Verification items for the finished model (mm, model axes). Coordinates: 2 decimals unless noted, no trailing zeros. Write each loop counter-clockwise with the first axis right and the second up, starting at its lowest first coordinate (ties: lowest second). Pieces come first, ordered by that corner, then holes. Notation, with made-up numbers: (33.5, 21) -> (51.5, 21) arc R17 ccw to (51.5, 48) -> close; hole circle Ø4 at (3.5, 85). An arc over 180 degrees is marked (long way). Answer in a Markdown table with one row per item.
```python
from build123d import *

# Parameters (mm, degrees)
SKETCH1_W               = 127
SKETCH1_H               = 101.6
BOSS_EXTRUDE1_DEPTH     = 3.175
CUT_EXTRUDE3_DEPTH      = 3.175
SKETCH4_W               = 6.35
SKETCH4_H               = 10.16
CUT_EXTRUDE4_DEPTH      = 3.175
MIRROR4_COPY_1_SKETCH_W = 6.35
MIRROR4_COPY_1_SKETCH_H = 10.16
MIRROR4_COPY_1_DEPTH    = 3.175


with BuildPart() as part:
    # Sketch1 → Boss-Extrude1 (new body)
    with BuildSketch(Plane(origin=(0, 0, 0), x_dir=(0, 0, -1), z_dir=(1, 0, 0))):
        Polygon((-127, -101.6), (-127, -155.575), (-114.3, -155.575), (-114.3, -152.4), (-101.6, -152.4), (-101.6, -155.575), (-88.9, -155.575), (-88.9, -152.4), (-76.2, -152.4), (-76.2, -155.575), (-63.5, -155.575), (-63.5, -101.6), (63.5, -101.6), (63.5, -155.575), (76.2, -155.575), (76.2, -152.4), (88.9, -152.4), (88.9, -155.575), (101.6, -155.575), (101.6, -152.4), (114.3, -152.4), (114.3, -155.575), (127, -155.575), (127, -101.6), (133.35, -101.6), (133.35, -50.8), (127, -50.8), (127, 50.8), (133.35, 50.8), (133.35, 101.6), (127, 101.6), (127, 155.575), (114.3, 155.575), (114.3, 152.4), (101.6, 152.4), (101.6, 155.575), (88.9, 155.575), (88.9, 152.4), (76.2, 152.4), (76.2, 155.575), (63.5, 155.575), (63.5, 101.6), (-63.5, 101.6), (-63.5, 155.575), (-76.2, 155.575), (-76.2, 152.4), (-88.9, 152.4), (-88.9, 155.575), (-101.6, 155.575), (-101.6, 152.4), (-114.3, 152.4), (-114.3, 155.575), (-127, 155.575), (-127, 101.6), (-133.35, 101.6), (-133.35, 50.8), (-127, 50.8), (-127, -50.8), (-133.35, -50.8), (-133.35, -101.6), align=None)
        Rectangle(SKETCH1_W, SKETCH1_H, mode=Mode.SUBTRACT)
    extrude(amount=BOSS_EXTRUDE1_DEPTH)

    # Sketch3 → Cut-Extrude3 (cut)
    with BuildSketch(Plane(origin=(3.175, 0, 0), x_dir=(0, 0, -1), z_dir=(1, 0, 0))):
        with BuildLine():
            Line((1.060660172, 84.639339828), (0, 85.7))
            Line((0, 85.7), (-1.060660172, 84.639339828))
            ThreePointArc((-1.060660172, 84.639339828), (0, 84.2), (1.060660172, 84.639339828))
        make_face()
        with BuildLine():
            Line((-1.060660172, 84.639339828), (0, 85.7))
            Line((0, 85.7), (1.060660172, 84.639339828))
            ThreePointArc((1.060660172, 84.639339828), (1.385819299, 85.125974851), (1.5, 85.7))
            ThreePointArc((1.5, 85.7), (-0.574025149, 87.085819299), (-1.060660172, 84.639339828))
        make_face()
        with BuildLine():
            ThreePointArc((1.060660172, 67.760660172), (0, 68.2), (-1.060660172, 67.760660172))
            Line((-1.060660172, 67.760660172), (0, 66.7))
            Line((0, 66.7), (1.060660172, 67.760660172))
        make_face()
        with BuildLine():
            Line((0, 66.7), (-1.060660172, 67.760660172))
            ThreePointArc((-1.060660172, 67.760660172), (-0.574025149, 65.314180701), (1.5, 66.7))
            ThreePointArc((1.5, 66.7), (1.385819299, 67.274025149), (1.060660172, 67.760660172))
            Line((1.060660172, 67.760660172), (0, 66.7))
        make_face()
        with BuildLine():
            ThreePointArc((11, 76.2), (10.074025149, 77.585819299), (8.439339828, 77.260660172))
            Line((8.439339828, 77.260660172), (9.5, 76.2))
            Line((9.5, 76.2), (8.439339828, 75.139339828))
            ThreePointArc((8.439339828, 75.139339828), (10.074025149, 74.814180701), (11, 76.2))
        make_face()
        with BuildLine():
            Line((9.5, 76.2), (8.439339828, 77.260660172))
            ThreePointArc((8.439339828, 77.260660172), (8, 76.2), (8.439339828, 75.139339828))
            Line((8.439339828, 75.139339828), (9.5, 76.2))
        make_face()
        with BuildLine():
            ThreePointArc((-8, 76.2), (-8.114180701, 76.774025149), (-8.439339828, 77.260660172))
            Line((-8.439339828, 77.260660172), (-9.5, 76.2))
            Line((-9.5, 76.2), (-8.439339828, 75.139339828))
            ThreePointArc((-8.439339828, 75.139339828), (-8.114180701, 75.625974851), (-8, 76.2))
        make_face()
        with BuildLine():
            Line((-9.5, 76.2), (-8.439339828, 77.260660172))
            ThreePointArc((-8.439339828, 77.260660172), (-11, 76.2), (-8.439339828, 75.139339828))
            Line((-8.439339828, 75.139339828), (-9.5, 76.2))
        make_face()
    extrude(amount=-CUT_EXTRUDE3_DEPTH, mode=Mode.SUBTRACT)

    # Sketch4 → Cut-Extrude4 (cut)
    with BuildSketch(Plane(origin=(3.175, 0, 0), x_dir=(0, 0, -1), z_dir=(1, 0, 0))):
        with Locations((130.175, 86.36)):
            Rectangle(SKETCH4_W, SKETCH4_H)
        with Locations((130.175, 66.04)):
            Rectangle(SKETCH4_W, SKETCH4_H)
    cut_extrude4 = extrude(amount=-CUT_EXTRUDE4_DEPTH, mode=Mode.SUBTRACT)

    # Mirror3: Cut-Extrude4 across plane
    add(cut_extrude4.mirror(Plane.ZX), mode=Mode.SUBTRACT)

    # Mirror4: Cut-Extrude4 across plane
    add(cut_extrude4.mirror(Plane.XY), mode=Mode.SUBTRACT)

    # Mirror4 copy 1 sketch → Mirror4 copy 1 (cut)
    with BuildSketch(Plane(origin=(3.175, 0, 0), x_dir=(0, 0, 1), z_dir=(1, 0, 0))):
        with Locations((130.175, 86.36)):
            Rectangle(MIRROR4_COPY_1_SKETCH_W, MIRROR4_COPY_1_SKETCH_H)
        with Locations((130.175, 66.04)):
            Rectangle(MIRROR4_COPY_1_SKETCH_W, MIRROR4_COPY_1_SKETCH_H)
    extrude(amount=-MIRROR4_COPY_1_DEPTH, mode=Mode.SUBTRACT)


solid = part.part
```
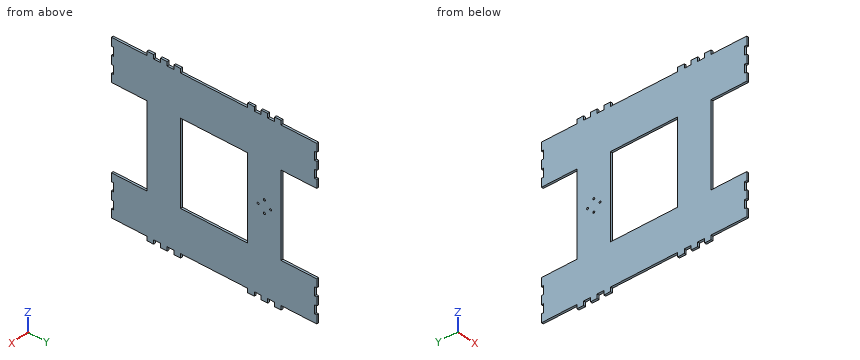
1. Go/stop test with flat-tipped pins: pin 1 (1 mm diameter, centred on x = 2, y = -133, fed in from +Z); pin 2 (1.6 mm diameter, centred on x = 2, y = -154.5, fed in from -Z); pin 3 (1 mm diameter, centred on x = 1.5, z = -79.5, fed in from -Y). Record where each tip stops, or that it passes through.
Findings below:
| item | result |
|---|---|
| pin 1 | stops at z = 127 |
| pin 2 | stops at z = -127 |
| pin 3 | stops at y = -152.4 |
2. Sectioned sample at B-B, the plane x = 1.4. Count the separate pieces of the cut face and the enclosed holes in it, and give its area (3 significant figures).
Findings below:
| item | result |
|---|---|
| separate pieces | 1 |
| enclosed holes | 5 |
| area | 52,800 mm² |
3. Material ranges on probe 1 along Y at (x, z) = (1.85, 9.5); probe 2 along Y at (x, z) = (1.85, 0); probe 3 along Z at (x, y) = (2.15, 76.2), recorded low to high. Write a range as from..to.
Findings below:
| item | result |
|---|---|
| probe 1 | y = -101.6..-50.8, 50.8..74.7, 77.7..101.6 |
| probe 2 | y = -101.6..-50.8, 50.8..65.2, 68.2..84.2, 87.2..101.6 |
| probe 3 | z = -133.35..-11, -8..8, 11..133.35 |
4. Sectioned sample at A-A, the plane y = 115. Record the cut outline in (x, z) (3 decimals).
Findings below:
| item | result |
|---|---|
| outline | (0, -127) -> (3.175, -127) -> (3.175, -63.5) -> (0, -63.5) -> close; (0, 63.5) -> (3.175, 63.5) -> (3.175, 127) -> (0, 127) -> close |
